Input: dimensioned drawing with shaded views. Units: mm. Origin: part minimum x, y, z. A direction names the side the tool comes from. Give positions to 0.01 mm unless a question says otherwise; leave off trailing zeros. Order: outer loops, then holes, each group sorted by start corner. A loop starts at its lowest first (then second) coordinate and runs counter-clockwise, first axis right, second up. Notation, with made-up numbers: (43.5, 43) - (68.5, 43) arc R13 cw to (68.5, 60) - close; hole circle Ø6 at (1.25, 85.25). An arc over 180 degrees is marked (long way). Answer as CSV lines item,"result".
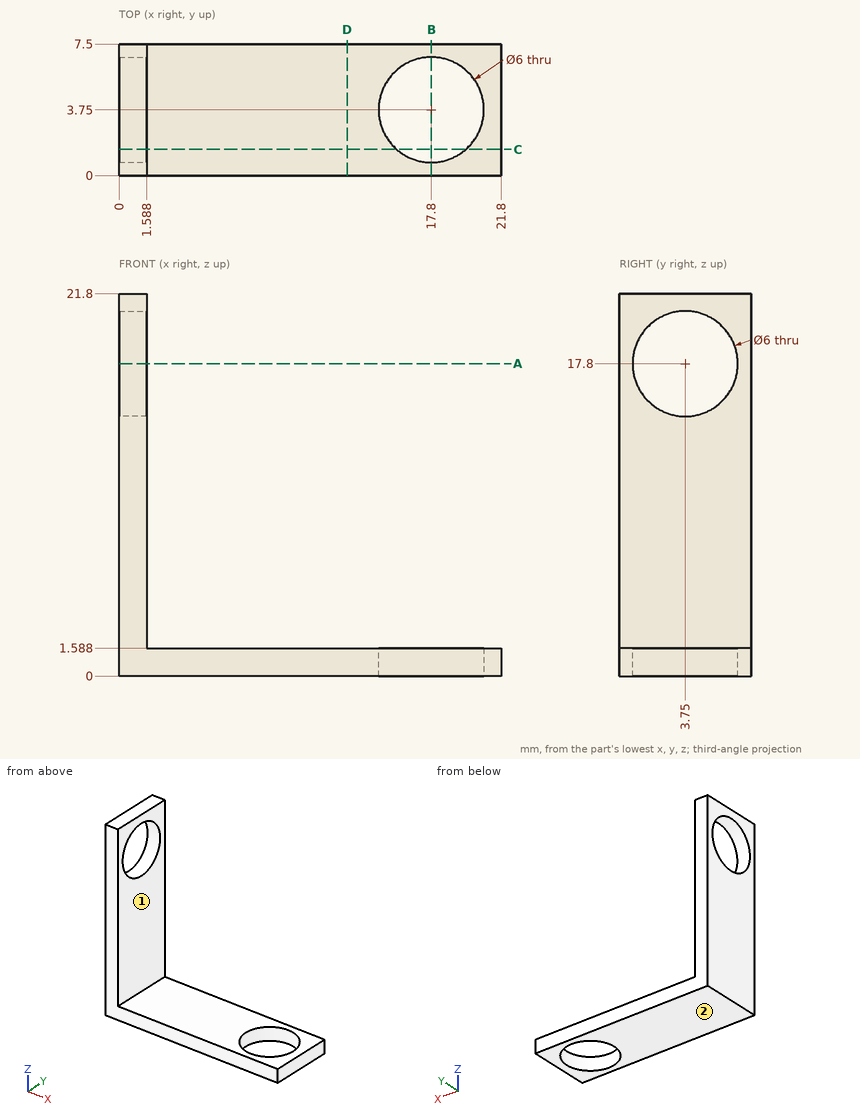
(1) Cut plane C-C (y = 1.5). Return loops of the section in (x, z) (1 decimal).
Completed:
outline,"(0, 0) - (15.8, 0) - (15.8, 1.6) - (1.6, 1.6) - (1.6, 15.8) - (0, 15.8) - close; (0, 19.8) - (1.6, 19.8) - (1.6, 21.8) - (0, 21.8) - close; (19.8, 0) - (21.8, 0) - (21.8, 1.6) - (19.8, 1.6) - close"
(2) Contact query for flat-ended pins moving along their axis: pin 1 (5 mm diameter, centred on x = 17.5, z = 4.5, fed in from -Y); pin 2 (4 mm diameter, centred on x = 11.5, y = 3, fed in from +Z); pin 3 (4 mm diameter, centred on y = 2, z = 10, fed in from +X). Output: stop coordinate, or through.
Completed:
pin 1,"through"
pin 2,"z = 1.59"
pin 3,"x = 1.59"
(3) Cut plane D-D (x = 13). Return loops of the section in (y, z).
Completed:
outline,"(0, 0) - (7.5, 0) - (7.5, 1.59) - (0, 1.59) - close"
(4) Cut plane A-A (z = 17.8). Return loops of the section in (x, y).
Completed:
outline,"(0, 0) - (1.59, 0) - (1.59, 0.75) - (0, 0.75) - close; (0, 6.75) - (1.59, 6.75) - (1.59, 7.5) - (0, 7.5) - close"
(5) Cut plane B-B (x = 17.8). Return loops of the section in (y, z).
Completed:
outline,"(0, 0) - (0.75, 0) - (0.75, 1.59) - (0, 1.59) - close; (6.75, 0) - (7.5, 0) - (7.5, 1.59) - (6.75, 1.59) - close"
(6) Ray query, line 1 (Y direction, x = 0.3, z = 17.8); line 2 (X direction, y = 1.5, z = 12). Return the intervals inside material, ascending. Write a range as from..to.
Completed:
line 1,"0..0.75, 6.75..7.5"
line 2,"0..1.59"
(7) Access query for the marked faces 1 and 2. Directions: +Z, -Z, +X, -X, +Y, -Y. A direction counts if a zero-diameter tool reaches every point of the face in a straight line with its end or side. Return the directions, or none.
Completed:
face 1,"+Z, +X, +Y, -Y"
face 2,"-Z, +X, -X, +Y, -Y"
